Autodesk Inventor part; units mm, degrees
ref_plane "YZ Plane" through (0, 0, 0) normal (1, 0, 0) x (0, 1, 0)
ref_plane "XZ Plane" through (0, 0, 0) normal (0, 1, 0) x (-1, 0, 0)
ref_plane "XY Plane" through (0, 0, 0) normal (0, 0, 1) x (1, 0, 0)
sketch "Sketch1" plane through (0, 0, 0) normal (0, 1, 0) x (-1, 0, 0)
  circle A0 centre (0, 0) radius 0.15
  dimension "d0" = 0.3
extrude "Extrusion1" add sketch "Sketch1" along normal blind 40
sketch "Sketch2" plane through (0, 40, 0) normal (0, 1, 0) x (1, 0, 0)
  circle A0 centre (0, 0) radius 0.5
  dimension "d3" = 1
extrude "Extrusion2" add sketch "Sketch2" along normal blind 33
sketch "Sketch3" plane through (0, 0, 0) normal (1, 0, 0) x (0, 1, 0)
  line L0 (73, -0.5) -> (73, 0.5)
  line L1 (73, 0) -> (73.4, 0)
  circle A0 centre (73.4, 0) radius 0.5
  point P0 (0, 0)
  dimension "d6" = 0.4
  dimension "d7" = 1
extrude "Extrusion3" add sketch "Sketch3" along normal mid plane 1.4
properties part number "neddle"
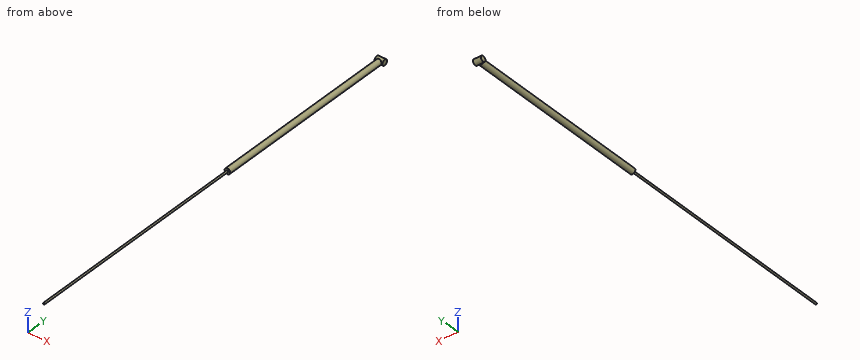
The listing builds one solid part. Answer for the finished solid, in the listing's coordinates (mm). Give positions to 0.01 mm unless a question says otherwise; leave off trailing zeros. Loops run counter-clockwise (first coordinate to the right, second up) from the corner with the lowest first, then second, coordinate; pieces in that order, holes last. Notation, with made-up numbers: (23, 6.5) - (64, 6.5) arc R15 ccw to (64, 20.5) - close; hole circle Ø8 at (13.5, 38.25). An arc over 180 degrees is marked (long way). Use one line per item in the form item = value.
1. Section B-B on y = 21 is taken. Give the vertices of the cut face in (x, z), then the cut area to 3 significant figures.
Calculated:
outline = circle Ø0.3 at (0, 0)
area = 0.0707 mm^2
2. Section C-C on y = 43 is taken. Give the vertices of the cut face in (x, z).
Calculated:
outline = circle Ø1 at (0, 0)
3. Section A-A on z = 0 is taken. Give the vertices of the cut face in (x, y).
Calculated:
outline = (-0.7, 72.9) - (-0.5, 72.9) - (-0.5, 40) - (-0.15, 40) - (-0.15, 0) - (0.15, 0) - (0.15, 40) - (0.5, 40) - (0.5, 72.9) - (0.7, 72.9) - (0.7, 73.9) - (-0.7, 73.9) - close
4. Find the intervals of material crossed by line 1 along Z through (x, y) = (0, 31); line 2 along X through (y, z) = (64, -0.1); line 3 along Z through (x, y) = (-0.4, 52), in increasing order. Write a range as [from, to].
Calculated:
line_1 = [-0.15, 0.15]
line_2 = [-0.49, 0.49]
line_3 = [-0.3, 0.3]
